For this review, take the finished solid that the model builds, in its own axes (mm). A direction names the side the tool comes from. Round coordinates to 2 decimals unless told otherwise and drop trailing zeros. Loops run counter-clockwise (first coordinate to the right, second up) from the corner with the lowest first, then second, coordinate; pieces in that order, holes last. Notation, with made-up numbers: (31.5, 88) -> (79.5, 88) arc R8 cw to (79.5, 93) -> close; hole circle Ø10 at (3, 72.5). An arc over 180 degrees is marked (long way). Write each question's results on one line, items separated by ' | '.
```python
from build123d import *

# Parameters (mm, degrees)
F0_R      = 8.5
F0_R_2    = 6.5
F1_DEPTH  = 23
F2_R      = 8.5
F3_DEPTH  = 2
F5_DEPTH  = 3
F6_R      = 2.99999
F7_R      = 2.75
F8_DEPTH  = 1.5
F9_R      = 3.35
F10_DEPTH = 2.5


# Not quite as in the source:
# - a fillet or chamfer that OpenCascade refuses, or shapes differently, is made with other operations: its cross-section is extruded or revolved along the edge and cut away or added
# - a fillet or chamfer is up to 0.001 mm smaller than in the source, because OpenCascade refuses the exact size


with BuildPart() as f1:
    # F0 (on Top) → F1 (new body)
    with BuildSketch(Plane.XY):
        Circle(F0_R)
        Circle(F0_R_2, mode=Mode.SUBTRACT)
    extrude(amount=F1_DEPTH)

    # F2 (on face) → F3 (join)
    with BuildSketch(Plane.XY.offset(23)):
        Circle(F2_R)
    extrude(amount=F3_DEPTH)

    # F4 (on face) → F5 (join)
    with BuildSketch(Plane(origin=(0, 0, 0), x_dir=(1, 0, 0), z_dir=(0, 0, -1))):
        with BuildLine():
            ThreePointArc((-5.5, 6.4807406984), (-2.9294798227, 7.9792322919), (0, 8.5))
            Line((0, 8.5), (0, 12))
            Line((0, 12), (-5.5, 12))
            Line((-5.5, 12), (-5.5, 6.4807406984))
        make_face()
        with BuildLine():
            Line((0, 12), (0, 8.5))
            ThreePointArc((0, 8.5), (2.9294798227, 7.9792322919), (5.5, 6.4807406984))
            Line((5.5, 6.4807406984), (5.5, 12))
            Line((5.5, 12), (0, 12))
        make_face()
    extrude(amount=-F5_DEPTH)

    # F6 (radius 3 in the source; OpenCascade refuses exactly that, so slightly less here)
    f6_edges = [f1.edges().sort_by_distance(p)[0] for p in [
        (0, -12, 0),
    ]]
    fillet(f6_edges, radius=F6_R)

    # F7 (on face) → F8 (join)
    with BuildSketch(Plane.XY.offset(25)):
        Circle(F7_R)
    extrude(amount=F8_DEPTH)

    # F9 (on face) → F10 (join)
    with BuildSketch(Plane.XY.offset(26.5)):
        Circle(F9_R)
    extrude(amount=F10_DEPTH)

    # F11: fillet of radius 3 on 1 edges, made by hand

    # F11_s1 → F11_t2 (revolve, cut)
    with BuildSketch(Plane.XZ):
        with BuildLine():
            ThreePointArc((3.35, 26.5), (2.3284517816, 28.2912878475), (0.3919601084, 29))
            Line((0.3919601084, 29), (3.35, 29))
            Line((3.35, 29), (3.35, 26.5))
        make_face()
    revolve(axis=Axis((0, 0, 29), (0, 0, 1)), mode=Mode.SUBTRACT)


solid = f1.part
```
1. Draft analysis for pull direction Y (two halves, no side actions). For faces 1 (the face through (0, 0, 23)), 2 (the face through (-0.596, -2.685, 25.74)), 3 (the face through (0, 3, 26.5)), state which applies: released by +Y, released by -Y, zero draft, split by the parting line, or undercut.
Values found:
face 1: undercut | face 2: split by the parting line | face 3: zero draft
2. Consider section C-C (y = -5.25). State the section outline as (x, z) points.
Values found:
outline: (-6.68, 0) -> (-3.83, 0) -> (-3.83, 23) -> (3.83, 23) -> (3.83, 0) -> (6.68, 0) -> (6.68, 25) -> (-6.68, 25) -> close
3. Tool access review of faces 4 (the face through (-5.5, -9, 1)), 5 (the face through (-5.158, -3.955, 11.339)), 6 (the face through (5.5, -9, 1)), 7 (the face through (-1.107, 8.428, 12.325)): name each direction out of +Z, -Z, +X, -X, +Y, -Y from which nothing blocks a thin tool from reaching the whole face with its end or side.
Values found:
face 4: +Z, -Z, -X, -Y | face 5: -Z | face 6: +Z, -Z, +X, -Y | face 7: +Z
4. To check wall thickness, follow probe 1 along Y at (x, z) = (0, 11); probe 2 along Z at (x, y) = (-5, -7.5); probe 3 along Z at (x, y) = (-4, -6.75). State the ranges of each line that lie inside material, in increasing order.
Values found:
probe 1: y = -8.5 to -6.5, 6.5 to 8.5 | probe 2: z = 0 to 3 | probe 3: z = 0 to 25
5. Consider section A-A (z = 14.25). State the section outline as (x, y) points, plus the area to 3 significant figures.
Values found:
outline: circle Ø17 at (0, 0); hole circle Ø13 at (0, 0) | area: 94.2 mm2
6. For pin 1 (2 mm diameter, centred on y = -2.5, z = 25, fed in from +X); pin 2 (5.5 mm diameter, centred on x = 1, y = -1.5, fed in from -Z); pin 3 (1.5 mm diameter, centred on y = 3, z = 3, fed in from -X), all flat-tipped, find the tip position at first contact; note any pin that passes through.
Values found:
pin 1: stops at x = 8.37 | pin 2: stops at z = 23 | pin 3: stops at x = -8.2
7. Consider section D-D (z = 23.5). State the section outline as (x, y) points.
Values found:
outline: circle Ø17 at (0, 0)
